Here's how the part is built. I have some questions about the finished solid (model axes, mm). A direction names the side the tool comes from. Coordinates: 2 decimals unless noted, no trailing zeros. Loops run counter-clockwise (first coordinate to the right, second up) from the corner with the lowest first, then second, coordinate; pieces in that order, holes last.
```python
from build123d import *

# Parameters (mm, degrees)
COUPLING_BARREL_SKETCH_R         = 6
COUPLING_BARREL_DEPTH            = 20
SERVICE_LOCK_DISC_SKETCH_R       = 12
SERVICE_LOCK_DISC_DEPTH          = 3
SHAFT_RUNNING_BORE_SKETCH_R      = 3.05
SHAFT_RUNNING_BORE_DEPTH         = 20.2
TORQUE_CROSS_PIN_HOLE_1_SKETCH_R = 1
TORQUE_CROSS_PIN_HOLE_1_DEPTH    = 26
TORQUE_CROSS_PIN_HOLE_2_SKETCH_R = 1
TORQUE_CROSS_PIN_HOLE_2_DEPTH    = 26
SERVICE_LOCK_POSITION_1_SKETCH_R = 1.6
SERVICE_LOCK_POSITION_1_DEPTH    = 3.2
SERVICE_LOCK_POSITION_2_SKETCH_R = 1.6
SERVICE_LOCK_POSITION_2_DEPTH    = 3.2
SERVICE_LOCK_POSITION_3_SKETCH_R = 1.6
SERVICE_LOCK_POSITION_3_DEPTH    = 3.2
SERVICE_LOCK_POSITION_4_SKETCH_R = 1.6
SERVICE_LOCK_POSITION_4_DEPTH    = 3.2
SERVICE_LOCK_POSITION_5_SKETCH_R = 1.6
SERVICE_LOCK_POSITION_5_DEPTH    = 3.2
SERVICE_LOCK_POSITION_6_SKETCH_R = 1.6
SERVICE_LOCK_POSITION_6_DEPTH    = 3.2
SERVICE_LOCK_POSITION_7_SKETCH_R = 1.6
SERVICE_LOCK_POSITION_7_DEPTH    = 3.2
SERVICE_LOCK_POSITION_8_SKETCH_R = 1.6
SERVICE_LOCK_POSITION_8_DEPTH    = 3.2


with BuildPart() as part:
    # Coupling barrel sketch → Coupling barrel (new body)
    with BuildSketch(Plane(origin=(-7, 0, 0), x_dir=(0, 0, -1), z_dir=(1, 0, 0))):
        with Locations((19.5, -29)):
            Circle(COUPLING_BARREL_SKETCH_R)
    extrude(amount=COUPLING_BARREL_DEPTH)

    # Service lock disc sketch → Service lock disc (add)
    with BuildSketch(Plane(origin=(-7, 0, 0), x_dir=(0, 0, -1), z_dir=(1, 0, 0))):
        with Locations((19.5, -29)):
            Circle(SERVICE_LOCK_DISC_SKETCH_R)
    extrude(amount=SERVICE_LOCK_DISC_DEPTH)

    # Shaft running bore sketch → Shaft running bore (cut)
    with BuildSketch(Plane(origin=(-7.1, 0, 0), x_dir=(0, 0, -1), z_dir=(1, 0, 0))):
        with Locations((19.5, -29)):
            Circle(SHAFT_RUNNING_BORE_SKETCH_R)
    extrude(amount=SHAFT_RUNNING_BORE_DEPTH, mode=Mode.SUBTRACT)

    # Torque cross pin hole 1 sketch → Torque cross pin hole 1 (cut)
    with BuildSketch(Plane(origin=(0, -42, 0), x_dir=(1, 0, 0), z_dir=(0, 1, 0))):
        with Locations(Location((-2, 19.5, 0), (0, 0, 90))):
            Circle(TORQUE_CROSS_PIN_HOLE_1_SKETCH_R)
    extrude(amount=TORQUE_CROSS_PIN_HOLE_1_DEPTH, mode=Mode.SUBTRACT)

    # Torque cross pin hole 2 sketch → Torque cross pin hole 2 (cut)
    with BuildSketch(Plane(origin=(0, -42, 0), x_dir=(1, 0, 0), z_dir=(0, 1, 0))):
        with Locations(Location((9, 19.5, 0), (0, 0, 90))):
            Circle(TORQUE_CROSS_PIN_HOLE_2_SKETCH_R)
    extrude(amount=TORQUE_CROSS_PIN_HOLE_2_DEPTH, mode=Mode.SUBTRACT)

    # Service lock position 1 sketch → Service lock position 1 (cut)
    with BuildSketch(Plane(origin=(-7.1, 0, 0), x_dir=(0, 0, -1), z_dir=(1, 0, 0))):
        with Locations((19.5, -20)):
            Circle(SERVICE_LOCK_POSITION_1_SKETCH_R)
    extrude(amount=SERVICE_LOCK_POSITION_1_DEPTH, mode=Mode.SUBTRACT)

    # Service lock position 2 sketch → Service lock position 2 (cut)
    with BuildSketch(Plane(origin=(-7.1, 0, 0), x_dir=(0, 0, -1), z_dir=(1, 0, 0))):
        with Locations((13.136038969, -22.636038969)):
            Circle(SERVICE_LOCK_POSITION_2_SKETCH_R)
    extrude(amount=SERVICE_LOCK_POSITION_2_DEPTH, mode=Mode.SUBTRACT)

    # Service lock position 3 sketch → Service lock position 3 (cut)
    with BuildSketch(Plane(origin=(-7.1, 0, 0), x_dir=(0, 0, -1), z_dir=(1, 0, 0))):
        with Locations((10.5, -29)):
            Circle(SERVICE_LOCK_POSITION_3_SKETCH_R)
    extrude(amount=SERVICE_LOCK_POSITION_3_DEPTH, mode=Mode.SUBTRACT)

    # Service lock position 4 sketch → Service lock position 4 (cut)
    with BuildSketch(Plane(origin=(-7.1, 0, 0), x_dir=(0, 0, -1), z_dir=(1, 0, 0))):
        with Locations((13.136038969, -35.363961031)):
            Circle(SERVICE_LOCK_POSITION_4_SKETCH_R)
    extrude(amount=SERVICE_LOCK_POSITION_4_DEPTH, mode=Mode.SUBTRACT)

    # Service lock position 5 sketch → Service lock position 5 (cut)
    with BuildSketch(Plane(origin=(-7.1, 0, 0), x_dir=(0, 0, -1), z_dir=(1, 0, 0))):
        with Locations((19.5, -38)):
            Circle(SERVICE_LOCK_POSITION_5_SKETCH_R)
    extrude(amount=SERVICE_LOCK_POSITION_5_DEPTH, mode=Mode.SUBTRACT)

    # Service lock position 6 sketch → Service lock position 6 (cut)
    with BuildSketch(Plane(origin=(-7.1, 0, 0), x_dir=(0, 0, -1), z_dir=(1, 0, 0))):
        with Locations((25.863961031, -35.363961031)):
            Circle(SERVICE_LOCK_POSITION_6_SKETCH_R)
    extrude(amount=SERVICE_LOCK_POSITION_6_DEPTH, mode=Mode.SUBTRACT)

    # Service lock position 7 sketch → Service lock position 7 (cut)
    with BuildSketch(Plane(origin=(-7.1, 0, 0), x_dir=(0, 0, -1), z_dir=(1, 0, 0))):
        with Locations((28.5, -29)):
            Circle(SERVICE_LOCK_POSITION_7_SKETCH_R)
    extrude(amount=SERVICE_LOCK_POSITION_7_DEPTH, mode=Mode.SUBTRACT)

    # Service lock position 8 sketch → Service lock position 8 (cut)
    with BuildSketch(Plane(origin=(-7.1, 0, 0), x_dir=(0, 0, -1), z_dir=(1, 0, 0))):
        with Locations((25.863961031, -22.636038969)):
            Circle(SERVICE_LOCK_POSITION_8_SKETCH_R)
    extrude(amount=SERVICE_LOCK_POSITION_8_DEPTH, mode=Mode.SUBTRACT)


solid = part.part
```
1. I need wall thicknesses on line 1 along X through (y, z) = (-24.35, -19.5); line 2 along Y through (x, z) = (-6.1, -19.5); line 3 along Y through (x, z) = (-5.75, -11.75). Which ranges of each line are inside material? Lowest first, please.
2. I want a section at D-D (x = -2). Please give me the cut outline in (y, z), then the cut area to 3 significant figures.
3. We'd pull the mould along X, two halves only. Please class faces 3 (the cylindrical face through (-5.52, -17.1, -17.94)), 4 (the cylindrical face through (8.01, -33.46, -19.37)), 5 (the flat face through (13, -26, -18)): +X half, -X half, draft (parallel to the pull), parting line (faces both ways), or undercut.
4. On a 3-axis mill with a long thin cutter (end or side, diameter ignored), from which of +Z, -Z, +X, -X, +Y, -Y can I reach the whole of each face in a straight line? I mean faces 1 (the cylindrical face through (4.381, -34.323, -22.269)), 2 (the cylindrical face through (-5.5, -24.2, -12.8)). Say none if no direction works.
5. I want a section at A-A (y = -28.5). Please give me the cut outline in (x, z).
6. I want a section at B-B (z = -17.5). Please give me the cut outline in (x, y).
7. For pin 1 (5 mm diameter, centred on y = -22.64, z = -25.86, fed in from +X); pin 2 (10 mm diameter, centred on x = 9.5, z = -13.5, fed in from +Y); pin 3 (4 mm diameter, centred on x = 1, y = -24.5, fed in from +Z), each with a flat end and sliding along its axis, tell me the tip position at first contact or that it passes through.
8. I want a section at C-C (y = -22.25). Please give me the cut outline in (x, z), then the cut area to 3 significant figures.
Response values:
1. line 1: x = -7 to -3, -1 to 8, 10 to 13
1. line 2: y = -41 to -39.6, -36.4 to -32.05, -25.95 to -21.6, -18.4 to -17
1. line 3: y = -38.16 to -36.16, -34.56 to -30, -28 to -23.44, -21.84 to -19.84
2. outline: (-34.92, -20.5) arc R6 ccw to (-23.08, -20.5) - (-26.12, -20.5) arc R3.05 cw to (-31.88, -20.5) - close; (-34.92, -18.5) - (-31.88, -18.5) arc R3.05 cw to (-26.12, -18.5) - (-23.08, -18.5) arc R6 ccw to start
2. area: 72.0 mm2
3. face 3: draft
3. face 4: undercut
3. face 5: +X half
4. face 1: +X
4. face 2: +X, -X
5. outline: (-7, -31.49) - (-4, -31.49) - (-4, -30.02) - (-7, -30.02) - close; (-7, -26.98) - (-4, -26.98) - (-4, -25.48) - (13, -25.48) - (13, -22.51) - (-7, -22.51) - close; (-7, -16.49) - (13, -16.49) - (13, -13.52) - (-4, -13.52) - (-4, -12.02) - (-7, -12.02) - close; (-7, -8.98) - (-4, -8.98) - (-4, -7.51) - (-7, -7.51) - close
6. outline: (-7, -40.83) - (-4, -40.83) - (-4, -34.66) - (13, -34.66) - (13, -31.3) - (-7, -31.3) - close; (-7, -26.7) - (13, -26.7) - (13, -23.34) - (-4, -23.34) - (-4, -17.17) - (-7, -17.17) - close
7. pin 1: stops at x = -4
7. pin 2: stops at y = -23.08
7. pin 3: stops at z = -14.05
8. outline: (-7, -29.42) - (-4, -29.42) - (-4, -27.42) - (-7, -27.42) - close; (-7, -24.31) - (-4, -24.31) - (-4, -14.69) - (-7, -14.69) - close; (-7, -11.58) - (-4, -11.58) - (-4, -9.58) - (-7, -9.58) - close
8. area: 40.9 mm2
